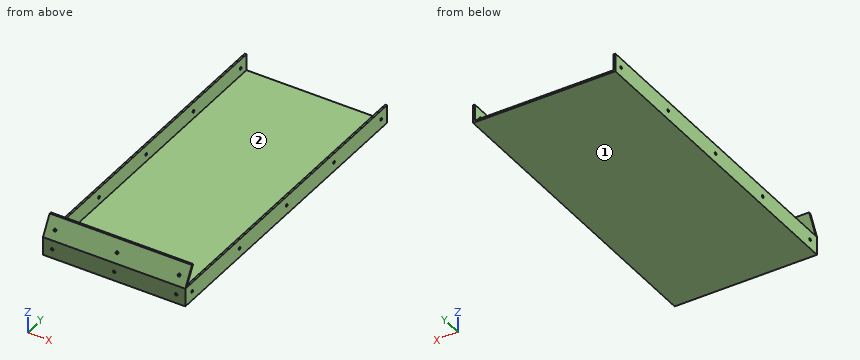
```python
from build123d import *

# Parameters (mm, degrees)
SKETCH057_W     = 156
SKETCH057_H     = 40
PAD017_DEPTH    = 350
POCKET035_DEPTH = 156.001
SKETCH059_R     = 1.5
POCKET036_DEPTH = 5
SKETCH060_R     = 1.5
POCKET037_DEPTH = 5
SKETCH061_W     = 2
SKETCH061_H     = 18
PAD018_DEPTH    = 348
SKETCH062_R     = 1.5
POCKET038_DEPTH = 156.001


with BuildPart() as part:
    # Sketch057 (on Face1 of Binder015) → Pad017 (new body)
    with BuildSketch(Plane(origin=(0, -0.1, 0), x_dir=(-1, 0, 0), z_dir=(0, 1, 0))):
        with Locations((200, -203.2)):
            Rectangle(SKETCH057_W, SKETCH057_H)
    extrude(amount=PAD017_DEPTH)

    # Sketch058 (on Face4 of Binder015) → Pocket035 (cut, through all)
    with BuildSketch(Plane(origin=(-122, 0, 0), x_dir=(0, -1, 0), z_dir=(-1, 0, 0))):
        Polygon((-13.4470053838, -183.2), (-1.9, -203.2), (-1.9, -221.2), (-349.9, -221.2), (-349.9, -183.2), align=None)
        Polygon((0.1, -183.2), (-11.4470053838, -183.2), (0.1, -203.2), align=None)
    extrude(amount=POCKET035_DEPTH, mode=Mode.SUBTRACT)

    # Sketch059 (on Face6 of Pocket035) → Pocket036 (cut)
    with BuildSketch(Plane(origin=(0, 87.9131810245, -50.7566987298), x_dir=(1, 0, 0), z_dir=(0, -0.8660254038, 0.5))):
        with Locations((-200, -166.026362)):
            Circle(SKETCH059_R)
        with Locations((-268, -166.026362)):
            Circle(SKETCH059_R)
        with Locations((-132, -166.026362)):
            Circle(SKETCH059_R)
    extrude(amount=-POCKET036_DEPTH, mode=Mode.SUBTRACT)

    # Sketch060 (on Face4 of Pocket036) → Pocket037 (cut)
    with BuildSketch(Plane.XZ.offset(0.1)):
        with Locations((-200, -213.2)):
            Circle(SKETCH060_R)
        with Locations((-268, -213.2)):
            Circle(SKETCH060_R)
        with Locations((-132, -213.2)):
            Circle(SKETCH060_R)
    extrude(amount=-POCKET037_DEPTH, mode=Mode.SUBTRACT)

    # Sketch061 (on Face8 of Pocket037) → Pad018 (join)
    with BuildSketch(Plane(origin=(0, 1.9, 0), x_dir=(-1, 0, 0), z_dir=(0, 1, 0))):
        with Locations((277, -212.2)):
            Rectangle(SKETCH061_W, SKETCH061_H)
        with Locations((123, -212.2)):
            Rectangle(SKETCH061_W, SKETCH061_H)
    extrude(amount=PAD018_DEPTH)

    # Sketch062 (on Face18 of Pad018) → Pocket038 (cut, through all)
    with BuildSketch(Plane.YZ.offset(-122)):
        with Locations((257.9, -213.2)):
            Circle(SKETCH062_R)
        with Locations((339.9, -213.2)):
            Circle(SKETCH062_R)
        with Locations((175.9, -213.2)):
            Circle(SKETCH062_R)
        with Locations((93.9, -213.2)):
            Circle(SKETCH062_R)
        with Locations((11.9, -213.2)):
            Circle(SKETCH062_R)
    extrude(amount=-POCKET038_DEPTH, mode=Mode.SUBTRACT)


solid = part.part
```
Read the model definition and answer for the solid it produces. Units are mm, in the model's axes. Face numbers are marked on the shaded views. Give positions to 0.01 mm unless a question says otherwise; leave off trailing zeros. Order: outer loops, then holes, each group sorted by start corner. A loop starts at its lowest first (then second) coordinate and runs counter-clockwise, first axis right, second up. Notation, with made-up numbers: (52.25, -26) -> (111.25, -26) arc R27 ccw to (111.25, -8) -> close; hole circle Ø8 at (41, 70.25). An arc over 180 degrees is marked (long way). One line per item, written item: value. Start each with the question number.
(1) The part is cut by section B-B (z = -218). Determine the outline of the cut face in (x, y).
(2) For a pull along X with two mould halves and no side action, classify the marked faces 1 and 2 as released by +X, released by -X, zero draft, split by the parting line, or undercut.
(3) Straight lines are drawn through the part: L1, parallel to Y at x = -276.55, z = -213.2; L2, parallel to X at y = 56.5, z = -219; L3, parallel to Z at x = -213, y = 266. For each, find the intervals that lie inside material, in ascending order.
(4) The part is cut by section A-A (x = -158.5). Determine the outline of the cut face in (y, z), and give its area (3 significant figures).
(5) Flat-ended cylindrical pins translate along their axes: P1, Ø1, axis at x = -201.5, z = -216, coming from the +Y side; P2, Ø0.6, axis at x = -123.5, y = 221, coming from the +Z side; P3, Ø1.5, axis at x = -242.5, z = -196.5, coming from the -Y side. Find the tip coordinate at first contact, or state that the pin passes through.
Taken from the geometry:
1. outline: (-278, -0.1) -> (-122, -0.1) -> (-122, 349.9) -> (-124, 349.9) -> (-124, 1.9) -> (-276, 1.9) -> (-276, 349.9) -> (-278, 349.9) -> close
2. face 1: zero draft
2. face 2: undercut
3. L1: -0.1 to 10.4, 13.4 to 92.4, 95.4 to 174.4, 177.4 to 256.4, 259.4 to 338.4, 341.4 to 349.9
3. L2: -278 to -276, -124 to -122
3. L3: -223.2 to -221.2
4. outline: (-0.1, -223.2) -> (349.9, -223.2) -> (349.9, -221.2) -> (1.9, -221.2) -> (1.9, -203.2) -> (13.45, -183.2) -> (11.45, -183.2) -> (-0.1, -203.2) -> close
4. area: 776 mm^2
5. P1: y = 1.9
5. P2: z = -203.2
5. P3: y = 3.34
